Build history of the part. All positions in model axes, mm. A direction names the side the tool comes from. Round coordinates to 2 decimals unless told otherwise and drop trailing zeros. Order: outer loops, then holes, each group sorted by start corner. A loop starts at its lowest first (then second) coordinate and runs counter-clockwise, first axis right, second up. Notation, with made-up numbers: M 3,68.5 L 10,68.5 A24 ccw 10,107.5 Z; hole C 44,14 d8. An arc over 180 degrees is marked long. One line per item, written item: value. Start each with the question number.
Item 1: Band-saw the part on C-C, the plane z = -93.5. Write the cut outline in (x, y), then the cut area to 3 significant figures.
Item 2: Two-plate mould, pull along Z, no slides. Class faces 3 (the cylindrical face through (1.479, 196.735, 38.699)), 4 (the flat face through (0, 40, 33)), 5 (the cylindrical face through (1.479, 181.957, 36.105)): +Z half, -Z half, draft (parallel to the pull), parting line (faces both ways), or undercut.
Item 3: Pin check, flat tips, straight feed: pin 1 (1.5 mm diameter, centred on x = 1.5, z = -42.5, fed in from +Y); pin 2 (1.5 mm diameter, centred on x = 2, y = 148, fed in from -Z); pin 3 (0.9 mm diameter, centred on x = 2, z = -77.5, fed in from +Y). Stop position of each tip, or through.
Item 4: Probe L1, parallel to Z at x = 2.2, y = 152; L2, parallel to Z at x = 1.65, y = 105; L3, parallel to Y at x = 1.45, z = 91. List the from-to ranges inside material, lowest first.
Item 5: Band-saw the part on B-B, the plane y = 115. Write the cut outline in (x, z), then the cut area to 3 significant figures.
Item 6: Band-saw the part on D-D, the plane x = 1.1. Give the number of separate pieces and of enclosed holes in the cut face, then the cut area to 3 significant figures.
Item 7: Band-saw the part on A-A, the plane z = 78.5. Write the cut outline in (x, y).
Item 8: Tool access for faces 1 (the flat face through (1.5, 91.4, 15.5)), 2 (the flat face through (1.48, 108.87, -5.42)): list every direction of +Z, -Z, +X, -X, +Y, -Y with a clear straight run to the whole face (end or side of a thin tool).
```python
from build123d import *

# Parameters (mm, degrees)
BOSS_EXTRUDE1_DEPTH     = 3
SKETCH2_W               = 27.727272727
SKETCH2_H               = 3
SKETCH2_W_2             = 3
SKETCH2_H_2             = 18
SKETCH2_H_3             = 9
SKETCH2_W_3             = 23.343342349
SKETCH2_W_4             = 23.34334235
SKETCH2_W_5             = 6
CUT_EXTRUDE1_DEPTH      = 1
CUT_EXTRUDE1_DEPTH_BACK = 4
SKETCH3_W               = 3.2
SKETCH3_H               = 10.5
SKETCH3_W_2             = 5.2
SKETCH3_H_2             = 2.5
CUT_EXTRUDE2_DEPTH      = 1
CUT_EXTRUDE2_DEPTH_BACK = 4
FILLET1_R               = 2.5
SKETCH4_R               = 5
BOSS_EXTRUDE2_DEPTH     = 3
FILLET2_R               = 2.5
SKETCH5_R               = 2.5
SKETCH5_R_2             = 2
SKETCH5_W               = 3.05
SKETCH5_H               = 15
CUT_EXTRUDE3_DEPTH      = 1
CUT_EXTRUDE3_DEPTH_BACK = 4


with BuildPart() as part:
    # Sketch1 → Boss-Extrude1 (new body)
    with BuildSketch(Plane(origin=(0, 0, 0), x_dir=(0, 0, -1), z_dir=(1, 0, 0))):
        with BuildLine():
            Line((-152.5, 33), (152.5, 33))
            Line((152.5, 33), (152.5, 23))
            Line((152.5, 23), (107.5, 23))
            ThreePointArc((107.5, 23), (72.144660941, 8.355339059), (57.5, -27))
            Line((57.5, -27), (57.5, -33))
            Line((57.5, -33), (-152.5, -33))
            Line((-152.5, -33), (-152.5, 33))
        make_face()
    extrude(amount=BOSS_EXTRUDE1_DEPTH)

    # Sketch2 → Cut-Extrude1 (cut, two sides)
    with BuildSketch(Plane(origin=(3, 0, 0), x_dir=(0, 0, -1), z_dir=(1, 0, 0))) as cut_extrude1_sk:
        with Locations((27.727272728, 31.5)):
            Rectangle(SKETCH2_W, SKETCH2_H)
        with Locations((83.181818182, 31.5)):
            Rectangle(SKETCH2_W, SKETCH2_H)
        with Locations((-138.636363636, 31.5)):
            Rectangle(SKETCH2_W, SKETCH2_H)
        with Locations((-83.181818182, 31.5)):
            Rectangle(SKETCH2_W, SKETCH2_H)
        with Locations((-27.727272728, 31.5)):
            Rectangle(SKETCH2_W, SKETCH2_H)
        with Locations((-151, 3)):
            Rectangle(SKETCH2_W_2, SKETCH2_H_2)
        with Locations((-151, -28.5)):
            Rectangle(SKETCH2_W_2, SKETCH2_H_3)
        with Locations((-117.484986475, -28.5)):
            Rectangle(SKETCH2_W_3, SKETCH2_H)
        with Locations((-70.798301777, -28.5)):
            Rectangle(SKETCH2_W_3, SKETCH2_H)
        with Locations((22.575067622, -28.5)):
            Rectangle(SKETCH2_W_4, SKETCH2_H)
        with Locations((149.5, 31.5)):
            Rectangle(SKETCH2_W_5, SKETCH2_H)
        with Locations((-24.111617078, -28.5)):
            Rectangle(SKETCH2_W_3, SKETCH2_H)
    extrude(amount=CUT_EXTRUDE1_DEPTH, mode=Mode.SUBTRACT)
    extrude(cut_extrude1_sk.sketch, amount=-CUT_EXTRUDE1_DEPTH_BACK, mode=Mode.SUBTRACT)

    # Sketch3 → Cut-Extrude2 (cut, two sides)
    with BuildSketch(Plane(origin=(3, 0, 0), x_dir=(0, 0, -1), z_dir=(1, 0, 0))) as cut_extrude2_sk:
        with Locations((-110.909090909, 27.75)):
            Rectangle(SKETCH3_W, SKETCH3_H)
        with Locations((55.454545455, 27.75)):
            Rectangle(SKETCH3_W, SKETCH3_H)
        with Locations((55.454545455, 28.575)):
            Rectangle(SKETCH3_W_2, SKETCH3_H_2)
        with Locations((-110.909090909, 28.575)):
            Rectangle(SKETCH3_W_2, SKETCH3_H_2)
    extrude(amount=CUT_EXTRUDE2_DEPTH, mode=Mode.SUBTRACT)
    extrude(cut_extrude2_sk.sketch, amount=-CUT_EXTRUDE2_DEPTH_BACK, mode=Mode.SUBTRACT)

    # Fillet1
    fillet1_edges = [part.edges().sort_by_distance(p)[0] for p in [
        (1.5, -33, -57.5),
    ]]
    fillet(fillet1_edges, radius=FILLET1_R)

    # Sketch4 → Boss-Extrude2 (add)
    with BuildSketch(Plane(origin=(0, 0, 0), x_dir=(0, 0, -1), z_dir=(1, 0, 0))):
        with BuildLine():
            Line((-55.454545455, 30), (-55.454545455, 177))
            ThreePointArc((-55.454545455, 177), (-38.304207087, 196.795944751), (-16.266602596, 182.641174423))
            Line((-16.266602596, 182.641174423), (27.727272727, 33))
            Line((27.727272727, 33), (27.727272727, 30))
            Line((27.727272727, 30), (-55.454545455, 30))
        make_face()
        with Locations((-35.454545455, 177)):
            Circle(SKETCH4_R, mode=Mode.SUBTRACT)
        Polygon((-30.454545455, 55), (-4.798665146, 55), (-30.454545455, 142.266148573), align=None, mode=Mode.SUBTRACT)
    extrude(amount=BOSS_EXTRUDE2_DEPTH)

    # Fillet2
    fillet2_edges = [part.edges().sort_by_distance(p)[0] for p in [
        (1.5, 55, 30.454545455),
        (1.5, 55, 4.798665146),
        (1.5, 142.266148573, 30.454545455),
    ]]
    fillet(fillet2_edges, radius=FILLET2_R)

    # Sketch5 → Cut-Extrude3 (cut, two sides)
    with BuildSketch(Plane(origin=(3, 0, 0), x_dir=(0, 0, -1), z_dir=(1, 0, 0))) as cut_extrude3_sk:
        with Locations((10.227172727, 31.5)):
            Circle(SKETCH5_R)
        with Locations((-35.454545455, 152)):
            Circle(SKETCH5_R)
        with Locations((-8.454545455, 46)):
            Circle(SKETCH5_R_2)
        Polygon((-3.003684653, 87.804874126), (-7.23456547, 102.195831269), (-4.308404184, 103.056110369), (-0.077523367, 88.665153225), align=None)
        with Locations((-42.954545455, 91.19961143)):
            Rectangle(SKETCH5_W, SKETCH5_H)
    extrude(amount=CUT_EXTRUDE3_DEPTH, mode=Mode.SUBTRACT)
    extrude(cut_extrude3_sk.sketch, amount=-CUT_EXTRUDE3_DEPTH_BACK, mode=Mode.SUBTRACT)


solid = part.part
```
Output:
1. outline: M 0,21 L 3,21 L 3,30 L 0,30 Z
1. area: 27.0 mm²
2. face 3: parting line
2. face 4: draft
2. face 5: undercut
3. pin 1: stops at y = 33
3. pin 2: stops at z = 5.86
3. pin 3: stops at y = 30
4. L1: z = 7.26 to 32.95, 37.95 to 55.45
4. L2: z = -6.56 to 19.5, 30.45 to 55.45
4. L3: y = -33 to 30
5. outline: M 0,-3.62 L 3,-3.62 L 3,22.44 L 0,22.44 Z; M 0,30.45 L 3,30.45 L 3,55.45 L 0,55.45 Z
5. area: 153 mm²
6. separate pieces: 1
6. enclosed holes: 11
6. area: 22,900 mm²
7. outline: M 0,-33 L 3,-33 L 3,-30 L 0,-30 Z; M 0,-27 L 3,-27 L 3,30 L 0,30 Z
8. face 1: +X, -X
8. face 2: -Z, +X, -X, +Y
